Read the model definition and answer for the solid it produces. Units are mm, in the model's axes. Face numbers are marked on the shaded views. A direction names the side the tool comes from. Give positions to 0.01 mm unless a question says otherwise; leave off trailing zeros. Write each loop counter-clockwise with the first axis right and the second up, starting at its lowest first coordinate (ties: lowest second). Pieces come first, ordered by that corner, then holes.
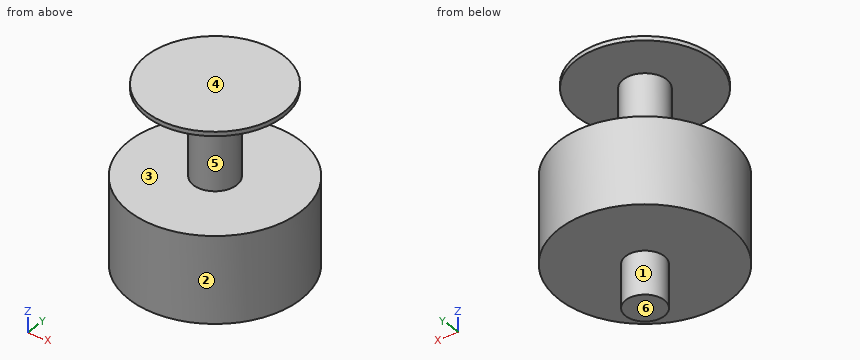
```python
from build123d import *

# Parameters (mm, degrees)
F0_R     = 12.7
F1_DEPTH = 12.7
F2_R     = 3.20606
F3_DEPTH = 12.7
F4_R     = 10.16
F5_DEPTH = 0.635
F6_R     = 2.86289
F7_DEPTH = 6.35


with BuildPart() as f1:
    # F0 (on Top) → F1 (new body)
    with BuildSketch(Plane.XY):
        Circle(F0_R)
    extrude(amount=F1_DEPTH)

    # F2 (on face) → F3 (join)
    with BuildSketch(Plane.XY.offset(12.7)):
        Circle(F2_R)
    extrude(amount=F3_DEPTH)

    # F4 (on face) → F5 (join)
    with BuildSketch(Plane.XY.offset(25.4)):
        Circle(F4_R)
    extrude(amount=F5_DEPTH)

    # F6 (on face) → F7 (join)
    with BuildSketch(Plane(origin=(0, 0, 0), x_dir=(1, 0, 0), z_dir=(0, 0, -1))):
        Circle(F6_R)
    extrude(amount=F7_DEPTH)


solid = f1.part
```
Item 1: Section D-D (y = -8.25) is taken. Write down the section's boundary in (x, z) (3 decimals), and give its area (3 significant figures).
Result set:
outline: (-9.655, 0) - (9.655, 0) - (9.655, 12.7) - (-9.655, 12.7) - close; (-5.93, 25.4) - (5.93, 25.4) - (5.93, 26.035) - (-5.93, 26.035) - close
area: 253 mm2
Item 2: Section A-A (x = 9) is taken. Write down the section's boundary in (y, z) (3 decimals).
Result set:
outline: (-8.96, 0) - (8.96, 0) - (8.96, 12.7) - (-8.96, 12.7) - close; (-4.714, 25.4) - (4.714, 25.4) - (4.714, 26.035) - (-4.714, 26.035) - close
Item 3: Section B-B (y = 0) is taken. Write down the section's boundary in (x, z) (3 decimals), and give its area (3 significant figures).
Result set:
outline: (-12.7, 0) - (-2.863, 0) - (-2.863, -6.35) - (2.863, -6.35) - (2.863, 0) - (12.7, 0) - (12.7, 12.7) - (3.206, 12.7) - (3.206, 25.4) - (10.16, 25.4) - (10.16, 26.035) - (-10.16, 26.035) - (-10.16, 25.4) - (-3.206, 25.4) - (-3.206, 12.7) - (-12.7, 12.7) - close
area: 453 mm2
Item 4: Determine the mould class of the marked faces 4, 5 and 6 for opening direction Z: pulls with the +Z half, pulls with the -Z half, needs draft (parallel to the pull), parting line crosses it, or undercut.
Result set:
face 4: pulls with the +Z half
face 5: undercut
face 6: pulls with the -Z half
Item 5: Find the intervals of material crossed by line 1 along Z through (x, y) = (7.25, 3.5) (3 decimals); line 2 along Z through (x, y) = (10.75, 0.75); line 3 along Z through (x, y) = (-1.75, 2.5) (3 decimals), in increasing order.
Result set:
line 1: z = 0 to 12.7, 25.4 to 26.035
line 2: z = 0 to 12.7
line 3: z = 0 to 26.035
Item 6: Each of these flat-tipped pins is pushed along its axis until it touches: pin 1 Ø2 at (x, y) = (-10, -2.5) entering from -Z; pin 2 Ø2 at (x, z) = (-3, 2) entering from -Y. Where does it stop, or does it pass through?
Result set:
pin 1: stops at z = 0
pin 2: stops at y = -12.54
Item 7: Which of the six approach directions +Z, -Z, +X, -X, +Y, -Y give full straight-line access (tool end or side, diameter ignored) to the marked faces 1, 2 and 3?
Result set:
face 1: -Z
face 2: +Z, -Z
face 3: none
